```python
from build123d import *

# Parameters (mm, degrees)
SKETCH1_R           = 53.614398493
SKETCH1_R_2         = 4
BOSS_EXTRUDE1_DEPTH = 16
SKETCH3_R           = 32
BOSS_EXTRUDE2_DEPTH = 6
SKETCH4_R           = 36
BOSS_EXTRUDE3_DEPTH = 18
BOSS_EXTRUDE4_START = 8
SKETCH5_R           = 32
BOSS_EXTRUDE4_DEPTH = 8
BOSS_EXTRUDE5_START = 24
SKETCH6_R           = 36
BOSS_EXTRUDE5_DEPTH = 24
FILLET2_R           = 4
CHAMFER2_SIZE       = 3
SKETCH7_R           = 24
CUT_EXTRUDE1_DEPTH  = 72


with BuildPart() as part:
    # Sketch1 → Boss-Extrude1 (new body)
    with BuildSketch(Plane(origin=(0, 0, 0), x_dir=(1, 0, 0), z_dir=(0, 1, 0))):
        with Locations(Location((0, 0, 0), (0, 0, 270))):
            Circle(SKETCH1_R)
        with Locations(Location((-44, 0, 0), (0, 0, 270))):
            Circle(SKETCH1_R_2, mode=Mode.SUBTRACT)
        with Locations(Location((-22, 38.105117767, 0), (0, 0, 270))):
            Circle(SKETCH1_R_2, mode=Mode.SUBTRACT)
        with Locations(Location((22, 38.105117767, 0), (0, 0, 270))):
            Circle(SKETCH1_R_2, mode=Mode.SUBTRACT)
        with Locations(Location((44, 0, 0), (0, 0, 270))):
            Circle(SKETCH1_R_2, mode=Mode.SUBTRACT)
        with Locations(Location((22, -38.105117767, 0), (0, 0, 270))):
            Circle(SKETCH1_R_2, mode=Mode.SUBTRACT)
        with Locations(Location((-22, -38.105117767, 0), (0, 0, 270))):
            Circle(SKETCH1_R_2, mode=Mode.SUBTRACT)
    extrude(amount=BOSS_EXTRUDE1_DEPTH)

    # Sketch3 → Boss-Extrude2 (add)
    with BuildSketch(Plane(origin=(0, 16, 0), x_dir=(1, 0, 0), z_dir=(0, 1, 0))):
        with Locations(Location((0, 0, 0), (0, 0, 270))):
            Circle(SKETCH3_R)
    extrude(amount=BOSS_EXTRUDE2_DEPTH)

    # Sketch4 → Boss-Extrude3 (add)
    with BuildSketch(Plane(origin=(0, 22, 0), x_dir=(1, 0, 0), z_dir=(0, 1, 0))):
        with Locations(Location((0, 0, 0), (0, 0, 270))):
            Circle(SKETCH4_R)
    extrude(amount=BOSS_EXTRUDE3_DEPTH)

    # Sketch5 → Boss-Extrude4 (add)
    with BuildSketch(Plane.XZ.offset(BOSS_EXTRUDE4_START)):
        with Locations(Location((0, 0, 0), (0, 0, 90))):
            Circle(SKETCH5_R)
    extrude(amount=-BOSS_EXTRUDE4_DEPTH)

    # Sketch6 → Boss-Extrude5 (add)
    with BuildSketch(Plane.XZ.offset(8).offset(BOSS_EXTRUDE5_START)):
        with Locations(Location((0, 0, 0), (0, 0, 90))):
            Circle(SKETCH6_R)
    extrude(amount=-BOSS_EXTRUDE5_DEPTH)

    # Fillet2
    fillet2_edges = [part.edges().sort_by_distance(p)[0] for p in [
        (0, 22, -32),
        (0, -8, -32),
    ]]
    fillet(fillet2_edges, radius=FILLET2_R - 0.0001)  # a hair under: the kernel refuses the full size

    # Chamfer2
    chamfer2_edges = [part.edges().sort_by_distance(p)[0] for p in [
        (0, 40, -36),
        (0, -32, -36),
    ]]
    chamfer(chamfer2_edges, length=CHAMFER2_SIZE)

    # Sketch7 → Cut-Extrude1 (cut)
    with BuildSketch(Plane(origin=(0, 40, 0), x_dir=(1, 0, 0), z_dir=(0, 1, 0))):
        with Locations(Location((0, 0, 0), (0, 0, 270))):
            Circle(SKETCH7_R)
    extrude(amount=-CUT_EXTRUDE1_DEPTH, mode=Mode.SUBTRACT)


solid = part.part
```
For this review, take the finished solid that the model builds, in its own axes (mm). A direction names the side the tool comes from. Round coordinates to 2 decimals unless told otherwise and drop trailing zeros. Write each loop counter-clockwise with the first axis right and the second up, starting at its lowest first coordinate (ties: lowest second). Pieces come first, ordered by that corner, then holes. Notation, with made-up numbers: (-25, 87.5) - (7, 87.5) arc R33 ccw to (7, 123.5) - close; hole circle Ø6 at (72.25, -31.5). An arc over 180 degrees is marked (long way). Answer as a JSON object with one key per item and string values.
1. To check wall thickness, follow line 1 along Y through (x, z) = (-6.5, 34.5); line 2 along Y through (x, z) = (-35, 36.5); line 3 along X through (y, z) = (23, -7). State the ranges of each line that lie inside material, in increasing order.
Response values:
{"line 1": "y = -29.89 to -7.9, 0 to 16, 21.9 to 37.89", "line 2": "y = 0 to 16", "line 3": "x = -35.31 to -22.96, 22.96 to 35.31"}
2. For pin 1 Ø1.5 at (x, y) = (-19, -13) entering from +Z; pin 2 Ø1.5 at (x, z) = (-31.5, 23) entering from -Y; pin 3 Ø8 at (x, y) = (12, -22) entering from -Z, all flat-tipped, find the tip position at first contact; note any pin that passes through.
Response values:
{"pin 1": "stops at z = 31.03", "pin 2": "stops at y = 0", "pin 3": "stops at z = -35.1"}
3. Draft analysis for pull direction Y (two halves, no side actions). For faces 1 (the face through (-31.24, 16.99, -6.94)), 2 (the face through (-20.169, 39.854, -26.303)), 3 (the face through (24.3, -32, 2.3)), 4 (the face through (24.703, 7.888, 35.157)), state which applies: +Y half, -Y half, draft (parallel to the pull), parting line (faces both ways), or undercut.
Response values:
{"face 1": "undercut", "face 2": "+Y half", "face 3": "-Y half", "face 4": "draft"}
4. Tool access review of faces 5 (the face through (-24.3, 40, 2.3)), 6 (the face through (-23, 0, 23)), 7 (the face through (-10.81, -18.65, 34.34)), 8 (the face through (10.81, 29.4, 34.34)), 9 (the face through (-19.297, 7.888, 35.157)): name each direction out of +Z, -Z, +X, -X, +Y, -Y from which nothing blocks a thin tool from reaching the whole face with its end or side.
Response values:
{"face 5": "+Z, -Z, +X, -X, +Y", "face 6": "none", "face 7": "-Y", "face 8": "+Y", "face 9": "+Y, -Y"}
5. We need section D-D on y = -22.5. Give the boundary of the cut face in (x, z).
Response values:
{"outline": "circle Ø72 at (0, 0); hole circle Ø48 at (0, 0)"}
6. We need section B-B on y = 7. Give the boundary of the cut face in (x, z), then the cut area to 3 significant figures.
Response values:
{"outline": "circle Ø107.23 at (0, 0); hole circle Ø8 at (-44, 0); hole circle Ø8 at (-22, -38.11); hole circle Ø8 at (-22, 38.11); hole circle Ø48 at (0, 0); hole circle Ø8 at (22, -38.11); hole circle Ø8 at (22, 38.11); hole circle Ø8 at (44, 0)", "area": "6,920 mm2"}
7. We need section C-C on z = 0. Count the separate pieces of the cut face and the enclosed holes in it, then the cut area to 3 significant figures.
Response values:
{"separate pieces": "4", "enclosed holes": "0", "area": "1,920 mm2"}
